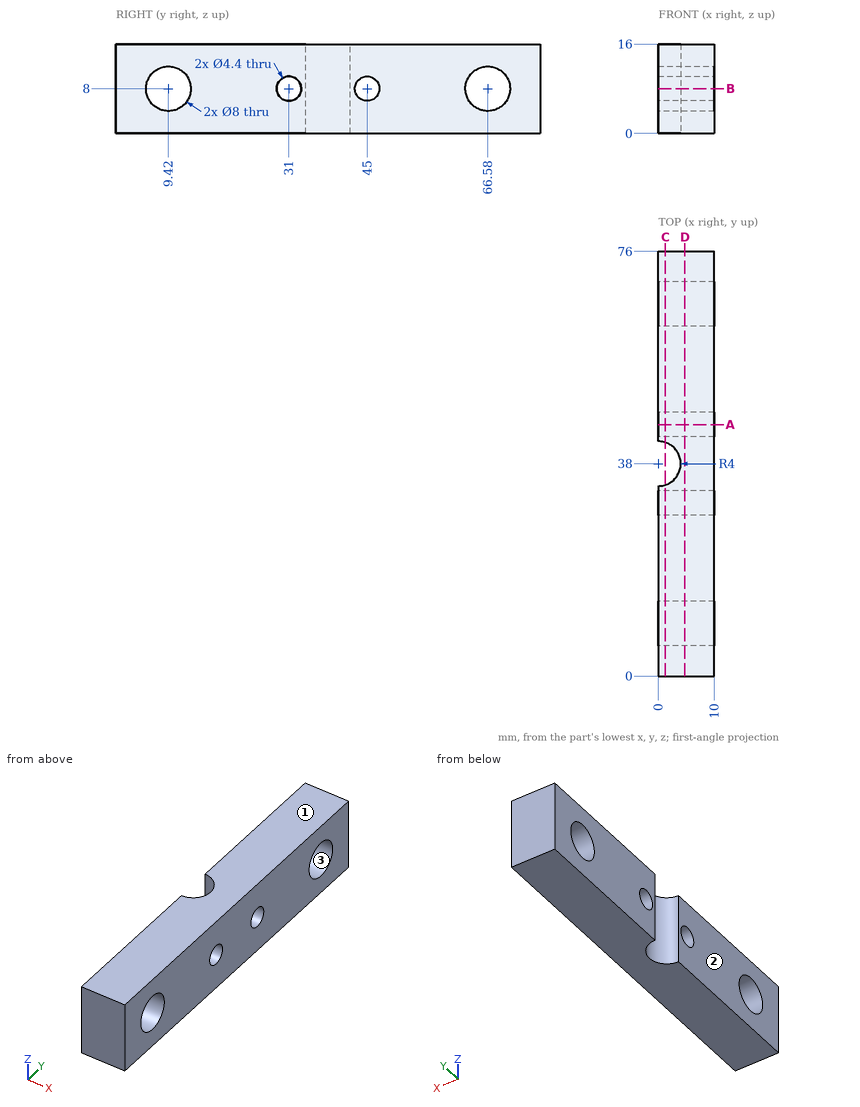
Source: three-view drawing plus pictorial views. Frame: mm from the lowest corner of the part. Coordinates: 2 decimals unless noted, no trailing zeros. Loops run counter-clockwise (first coordinate to the right, second up) from the corner with the lowest first, then second, coordinate; pieces in that order, holes last. Notation, with made-up numbers: (45, 84.5) -> (81, 84.5) arc R4 cw to (81, 90.5) -> close; hole circle Ø8 at (-40, -4). An arc over 180 degrees is marked (long way). Answer in a Markdown table with one row per item. Add a question column.
Q1. Section C-C on x = 1.25. Return the cut outline in (y, z), and give its area (3 significant figures).
Q2. Pull-direction query (Z, two-part tool) for the marked faces 1, 2 and 3; classes: pulls with the +Z half, pulls with the -Z half, needs draft (parallel to the pull), parting line crosses it, or undercut.
Q3. Section A-A on y = 45. Return the cut outline in (x, z).
Q4. Section B-B on z = 8. Return the cut outline in (x, y).
Q5. Section D-D on x = 4.75. Return the cut outline in (y, z).
Q6. Contact query for a flat-ended pin moving along its axis: pin 1 Ø2.5 at (y, z) = (31, 8) entering from -X. Output: stop coordinate, or through.
Q7. Ray query, line 1 along Y through (x, z) = (6.25, 8); line 2 along Z through (x, y) = (5.25, 31); line 3 along Y through (x, z) = (4.75, 7). Return the intervals inside material, ascending.
Computed values:
| question | item | result |
|---|---|---|
| 1 | outline | (0, 0) -> (34.2, 0) -> (34.2, 16) -> (0, 16) -> close; (41.8, 0) -> (76, 0) -> (76, 16) -> (41.8, 16) -> close; hole circle Ø8 at (9.42, 8); hole circle Ø4.4 at (31, 8); hole circle Ø4.4 at (45, 8); hole circle Ø8 at (66.58, 8) |
| 1 | area | 963 mm^2 |
| 2 | face 1 | pulls with the +Z half |
| 2 | face 2 | needs draft |
| 2 | face 3 | undercut |
| 3 | outline | (0, 0) -> (10, 0) -> (10, 5.8) -> (0, 5.8) -> close; (0, 10.2) -> (10, 10.2) -> (10, 16) -> (0, 16) -> close |
| 4 | outline | (0, 0) -> (10, 0) -> (10, 5.42) -> (0, 5.42) -> close; (0, 13.42) -> (10, 13.42) -> (10, 28.8) -> (0, 28.8) -> close; (0, 33.2) -> (10, 33.2) -> (10, 42.8) -> (0, 42.8) -> (0, 42) arc R4 cw to (0, 34) -> close; (0, 47.2) -> (10, 47.2) -> (10, 62.58) -> (0, 62.58) -> close; (0, 70.58) -> (10, 70.58) -> (10, 76) -> (0, 76) -> close |
| 5 | outline | (0, 0) -> (76, 0) -> (76, 16) -> (0, 16) -> close; hole circle Ø8 at (9.42, 8); hole circle Ø4.4 at (31, 8); hole circle Ø4.4 at (45, 8); hole circle Ø8 at (66.58, 8) |
| 6 | pin 1 | passes through |
| 7 | line 1 | y = 0 to 5.42, 13.42 to 28.8, 33.2 to 42.8, 47.2 to 62.58, 70.58 to 76 |
| 7 | line 2 | z = 0 to 5.8, 10.2 to 16 |
| 7 | line 3 | y = 0 to 5.55, 13.29 to 29.04, 32.96 to 43.04, 46.96 to 62.71, 70.45 to 76 |
